from build123d import *

# Parameters (mm, degrees)
F1_DEPTH = 34
F0_W     = 25.4
F0_H     = 1
F2_DEPTH = 25.4
F3_DEPTH = 7.9375
F5_R     = 4
F6_DEPTH = 16


with BuildPart() as f1:
    # F0 (on Front) → F1 (new body, symmetric)
    with BuildSketch(Plane.XZ):
        Polygon((40.275, 9.525), (-41.275, 9.525), (-41.275, -9.525), (41.275, -9.525), (41.275, 9.525), align=None)
    extrude(amount=F1_DEPTH, both=True)

    # F0 (on Front) → F2 (join, symmetric)
    with BuildSketch(Plane.XZ):
        with BuildLine():
            Line((40.275, 27.0002), (40.275, 9.525))
            Line((40.275, 9.525), (41.275, 9.525))
            Line((41.275, 9.525), (41.275, 27.0002))
            ThreePointArc((41.275, 27.0002), (45.9246798487, 38.2255201513), (57.15, 42.8752))
            Line((57.15, 42.8752), (60.325, 42.8752))
            Line((60.325, 42.8752), (60.325, 43.8752))
            Line((60.325, 43.8752), (57.15, 43.8752))
            add(Edge.make_bspline(
                [(55.9712612806, 43.8339815131), (56.3656474087, 43.8478093746), (56.7585819078, 43.8615403645), (57.15, 43.8752)],
                knots=[103.2345242702, 103.2345242702, 103.2345242702, 103.2345242702, 104.2469033835, 104.2469033835, 104.2469033835, 104.2469033835], degree=3))
            ThreePointArc((55.9712612806, 43.8339815131), (44.8078599731, 38.5083364502), (40.275, 27.0002))
        make_face()
        with Locations((73.025, 43.3752)):
            Rectangle(F0_W, F0_H)
    extrude(amount=F2_DEPTH, both=True)

    # F0 (on Front) → F3 (join, symmetric)
    with BuildSketch(Plane.XZ):
        with BuildLine():
            add(Edge.make_bspline(
                [(-41.275, 9.525), (-39.5560968864, 40.0065637522), (15.7548405948, 42.4239240696), (55.9712612806, 43.8339815131)],
                knots=[0, 0, 0, 0, 103.2345242702, 103.2345242702, 103.2345242702, 103.2345242702], degree=3))
            Line((-41.275, 9.525), (40.275, 9.525))
            Line((40.275, 9.525), (40.275, 27.0002))
            ThreePointArc((40.275, 27.0002), (44.8078599731, 38.5083364502), (55.9712612806, 43.8339815131))
        make_face()
    extrude(amount=F3_DEPTH, both=True)

    # F0 (on Front) → F4 (revolve)
    with BuildSketch(Plane.XZ):
        Polygon((85.725, 66.675), (85.725, 43.8752), (85.725, 42.8752), (85.725, 38.1), (111.125, 38.1), (111.125, 66.675), align=None)
    revolve(axis=Axis((85.725, 0, 52.3875), (0, 0, 1)))

    # F5
    f5_edges = [f1.edges().sort_by_distance(p)[0] for p in [
        (41.275, -34, 0),
        (-41.275, -34, 0),
        (41.275, 34, 0),
        (-41.275, 34, 0),
    ]]
    fillet(f5_edges, radius=F5_R)

    # F6 (add): a face of the model
    f6_faces = [f1.faces().sort_by_distance(p)[0] for p in [
        (85.725, 0, 66.675),
    ]]
    extrude(f6_faces, amount=-F6_DEPTH)


solid = f1.part
For this review, take the finished solid that the model builds, in its own axes (mm). A direction names the side the tool comes from. Round coordinates to 2 decimals unless told otherwise and drop trailing zeros. Order: outer loops, then holes, each group sorted by start corner. A loop starts at its lowest first (then second) coordinate and runs counter-clockwise, first axis right, second up. Notation, with made-up numbers: M 5.5,40.25 L 33.5,40.25 A18 ccw 33.5,72.25 Z; hole C 27.5,73.5 d4. An arc over 180 degrees is marked long. Use a Markdown table: item, result. Add a question column.
Item 1: Add section C-C, the plane x = 89.5. Give the boundary of the cut face in (y, z) (3 decimals).
Item 2: Add section B-B, the plane x = 71. Give the boundary of the cut face in (y, z) (3 decimals), then the cut area to 3 significant figures.
Item 3: Tool access review of faces 1 (the flat face through (51, 25.4, 42)), 2 (the flat face through (60, 2, 42.875)), 3 (the flat face through (60, -2, 43.875)): name each direction out of +Z, -Z, +X, -X, +Y, -Y from which nothing blocks a thin tool from reaching the whole face with its end or side.
Item 4: To check wall thickness, follow line 1 along X through (y, z) = (-16.5, 14) (3 decimals); line 2 along Z through (x, y) = (-24.5, 14.5) (3 decimals); line 3 along X through (y, z) = (13, 41.5). State the ranges of each line that lie inside material, in increasing order.
Item 5: Add section A-A, the plane z = 60.5. Give the boundary of the cut face in (x, y) (3 decimals).
Item 6: Insertion check: pin 1 (21 mm diameter, centred on x = -2.5, y = -24.5, fed in from +Z) (3 decimals); pin 2 (2 mm diameter, centred on y = 20, z = 58.5, fed in from +X); pin 3 (5 mm diameter, centred on y = 0, z = 24.5, fed in from -X). Each pin has a flat end and moves straight along its axis. Give the tip position at first contact, or say it passes through.
Geometry results:
| question | item | result |
|---|---|---|
| 1 | outline | M -25.118,38.1 L 25.118,38.1 L 25.118,66.675 L -25.118,66.675 Z |
| 2 | outline | M -25.4,42.875 L -20.696,42.875 L -20.696,38.1 L 20.696,38.1 L 20.696,42.875 L 25.4,42.875 L 25.4,43.875 L 20.696,43.875 L 20.696,66.675 L -20.696,66.675 L -20.696,43.875 L -25.4,43.875 Z |
| 2 | area | 1,190 mm² |
| 3 | face 1 | +Z, +X, -X, +Y |
| 3 | face 2 | -Z |
| 3 | face 3 | +Z, -X |
| 4 | line 1 | x = 40.275 to 41.275 |
| 4 | line 2 | z = -9.525 to 9.525 |
| 4 | line 3 | x = 48.52 to 50.69, 63.9 to 107.55 |
| 5 | outline | C 85.725,0 d50.8 |
| 6 | pin 1 | stops at z = 9.525 |
| 6 | pin 2 | stops at x = 102.58 |
| 6 | pin 3 | stops at x = -36.7 |
